Read the model definition and answer for the solid it produces. Units are mm, in the model's axes. Give positions to 0.01 mm unless a question says otherwise; leave off trailing zeros. Loops run counter-clockwise (first coordinate to the right, second up) from the corner with the lowest first, then second, coordinate; pieces in that order, holes last. Notation, with made-up numbers: (-5.75, 12.5) - (33.25, 12.5) arc R20 ccw to (33.25, 31.5) - close; hole circle Ø4 at (-35.5, 36). An arc over 180 degrees is marked (long way). Write item = value, one per line. Start each with the question number.
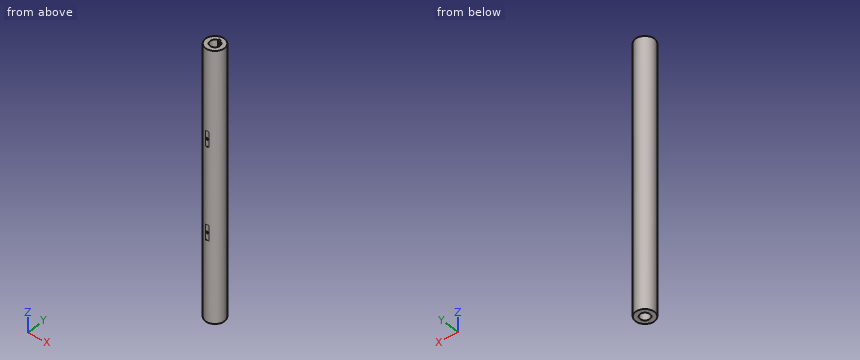
Autodesk Inventor part; units mm, degrees
ref_plane "YZ Plane" through (0, 0, 0) normal (1, 0, 0) x (0, 1, 0)
sketch "草图1" plane through (0, 0, 0) normal (0, 0, 1) x (1, 0, 0)
  circle A0 centre (0, 0) radius 12.5
  dimension "d0" = 25
extrude "拉伸1" add sketch "草图1" along normal mid plane 350
ref_plane "工作平面1" through (0, 0, 175) normal (0, 0, 1) x (1, 0, 0)
ref_plane "工作平面3" through (0, 0, -165) normal (0, 0, 1) x (1, 0, 0)
sketch "草图2" plane through (0, 0, 175) normal (0, 0, 1) x (1, 0, 0)
  circle A0 centre (0, 0) radius 6.5
  dimension "d64" = 13
sketch "草图3" plane through (0, 0, -165) normal (0, 0, 1) x (1, 0, 0)
  circle A0 centre (0, 0) radius 4.5
  circle A1 centre (0, 0) radius 6.5
  dimension "d15" = 9
  dimension "d16" = 13
extrude "拉伸2" cut sketch "草图3" along normal blind 350 contours A0
ref_plane "工作平面4" through (0, 12.5, 0) normal (0, 1, 0) x (-1, 0, 0)
sketch "草图8" plane through (0, 0, 175) normal (0, 0, 1) x (1, 0, 0)
  circle A0 centre (0, 0) radius 6.5
  circle A1 centre (0, 6.5) radius 1.5
  dimension "d37" = 3
ref_plane "工作平面5" through (0, -12.5, 0) normal (0, 1, 0) x (-1, 0, 0)
sketch "草图9" plane through (0, -12.5, 0) normal (0, 1, 0) x (-1, 0, 0)
  point P0 (0, 0)
  point P1 (0, 0)
  point P2 (0, 60)
  point P3 (0, -60)
  dimension "d41" = 60
  dimension "d42" = 60
hole "孔3" at (0, -12.5, 60) at (0, -12.5, -60) direction (0, 1, 0) diameter 2.459 depth 8.8 tip angle 118
ref_plane "工作平面6" through (0, 0, 60) normal (0, 0, 1) x (1, 0, 0)
sketch "草图11" plane through (0, 0, 60) normal (0, 0, 1) x (1, 0, 0)
  line L0 (0, 0) -> (0, -12.3)
  line L1 (2.2271, -12.3) -> (-2.2271, -12.3)
  arc A0 (2.2271, -12.3) -> (0, 12.5) centre (0, 0) ccw
  arc A1 (0, 12.5) -> (-2.2271, -12.3) centre (0, 0) ccw
  circle A2 centre (0, 0) radius 12.5
extrude "拉伸6" cut sketch "草图11" along normal mid plane 20 contours A2 L1
ref_plane "工作平面7" through (0, 0, -60) normal (0, 0, 1) x (1, 0, 0)
sketch "草图12" plane through (0, 0, -60) normal (0, 0, 1) x (1, 0, 0)
  line L0 (0, 0) -> (0, -12.3)
  line L1 (2.2271, -12.3) -> (-2.2271, -12.3)
  arc A0 (2.2271, -12.3) -> (0, 12.5) centre (0, 0) ccw
  arc A1 (0, 12.5) -> (-2.2271, -12.3) centre (0, 0) ccw
  circle A2 centre (0, 0) radius 12.5
extrude "拉伸7" cut sketch "草图12" along normal mid plane 20 contours A2 L1
ref_plane "工作平面8" through (0, 0, -175) normal (0, 0, 1) x (1, 0, 0)
sketch "草图13" plane through (0, 0, -175) normal (0, 0, 1) x (1, 0, 0)
  circle A0 centre (0, 0) radius 6.5
  dimension "d59" = 13
extrude "拉伸8" cut sketch "草图13" along normal blind 15
extrude "拉伸9" cut sketch "草图2" against normal blind 36
thread "螺纹3"
thread "螺纹5"
extrude "拉伸10" cut sketch "草图8" against normal blind 36 contours A1 A0 | A0 A1 picked at (0, 5.9871) picked at (-0.0289, 6.9863)
properties part number "殷钢管" material "钢，合金"
1. Consider line 1 along Y through (x, z) = (0, -58); line 2 along Y through (x, z) = (0, -168.25); line 3 along X through (y, z) = (1.5, 92). Determine where each line is inside the solid, lowest interval first. Write a range as [from, to].
2. A cutting plane is placed at B-B on z = -53. Give the vertices of the cut face in (x, y), and give its area (3 significant figures).
3. Given P1, Ø4, axis at x = 0, z = -60, coming from the -Y side; P2, Ø8, axis at y = -5.5, z = 60, coming from the -X side; P3, Ø6.5, axis at x = -1, y = 2, coming from the +Z side, each flat-ended and moving along its own axis, determine where each tip first touches the part or whether it passes through.
4. A cutting plane is placed at D-D on z = 91. Give the vertices of the cut face in (x, y).
5. A cutting plane is placed at C-C on z = 151.5. Give the vertices of the cut face in (x, y), and give its area (3 significant figures).
6. A cutting plane is placed at A-A on y = 0. Give the vertices of the cut face in (x, z).
Reply:
q1.line_1 = [-12.3, -4.5], [4.5, 12.5]
q1.line_2 = [-12.5, -6.5], [6.5, 12.5]
q1.line_3 = [-12.41, -4.24], [4.24, 12.41]
q2.outline = (-2.23, -12.3) - (2.23, -12.3) arc R12.5 ccw (long way) to start; hole circle Ø9 at (0, 0)
q2.area = 427 mm^2
q3.P1 = -12.3
q3.P2 = -12.41
q3.P3 = 139
q4.outline = circle Ø25 at (0, 0); hole circle Ø9 at (0, 0)
q5.outline = circle Ø25 at (0, 0); hole (-1.49, 6.33) arc R6.5 ccw (long way) to (1.49, 6.33) arc R1.5 ccw (long way) to start
q5.area = 354 mm^2
q6.outline = (-12.5, -175) - (-6.5, -175) - (-6.5, -160) - (-4.5, -160) - (-4.5, 139) - (-6.5, 139) - (-6.5, 175) - (-12.5, 175) - close; (4.5, -160) - (6.5, -160) - (6.5, -175) - (12.5, -175) - (12.5, 175) - (6.5, 175) - (6.5, 139) - (4.5, 139) - close
